Geometry check sheet. Reference: the model listing, model coordinates, mm. Face numbers are marked on the shaded views. A direction names the side the tool comes from. Round coordinates to 2 decimals unless told otherwise and drop trailing zeros. Write each loop counter-clockwise with the first axis right and the second up, starting at its lowest first coordinate (ties: lowest second). Pieces come first, ordered by that corner, then holes. Notation, with made-up numbers: M 54,78 L 89,78 A20 ccw 89,91 Z; hole C -27,-5.75 d10. An arc over 180 degrees is marked long. One line per item, written item: value. Start each with the question number.
1. Depth check by flat-ended pin: P1, Ø4, axis at x = 0, y = 8.5, coming from the +Z side; P2, Ø2, axis at y = 5.5, z = 36, coming from the -X side; P3, Ø0.5, axis at y = 4, z = 1.5, coming from the +X side. Enter the tip coordinate at first touch or a pass-through.
2. Scan lines: probe 1 along Y at (x, z) = (0, 1.2); probe 2 along Y at (x, z) = (-9, 29); probe 3 along X at (y, z) = (-9.25, 37). Record each from-to range of solid material in increasing order. Write a range as [from, to].
3. Section check D-D (z = 4). Record the boundary of the cut face in (x, y).
4. Release check for a two-part mould opening along Z. For the marked faces 4, 5, 6 and 7 record: pulls with the +Z half, pulls with the -Z half, needs draft (parallel to the pull), parting line crosses it, or undercut.
5. Section check A-A (x = 16.5). Record the boundary of the cut face in (y, z), and give its area (3 significant figures).
6. Access from +Z, -Z, +X, -X, +Y, -Y to the whole of each face (thin tool, end or side, straight path). Record for the marked faces 1, 2 and 3.
7. Section check B-B (y = 8.5). Count the separate pieces of the cut face and the enclosed holes in it, and give its area (3 significant figures).
8. Section check C-C (z = 44). Record the boundary of the cut face in (x, y), and give its area (3 significant figures).
from build123d import *

# Parameters (mm, degrees)
SKETCH1_R                = 14
BOSS_EXTRUDE1_DEPTH      = 50
SKETCH5_W                = 28
SKETCH5_H                = 50.034880911
BOSS_EXTRUDE2_DEPTH      = 21
SKETCH2_R                = 12.791811967
CUT_EXTRUDE1_DEPTH       = 48
SKETCH3_R                = 4
CUT_EXTRUDE2_DEPTH       = 49
SKETCH4_R                = 1.5
CUT_EXTRUDE3_DEPTH       = 49
SKETCH6_R                = 12.79
CUT_EXTRUDE5_DEPTH       = 21
SKETCH7_W                = 28
SKETCH7_H                = 4.634699127
CUT_EXTRUDE6_DEPTH       = 53
SKETCH8_W                = 50.034880911
SKETCH8_H                = 3.58
BOSS_EXTRUDE3_DEPTH      = 5
SKETCH13_R               = 1.5
CUT_EXTRUDE7_DEPTH       = 5
SKETCH14_W               = 50.034880911
SKETCH14_H               = 3.58
BOSS_EXTRUDE4_DEPTH      = 5
SKETCH15_R               = 1.5
CUT_EXTRUDE8_DEPTH       = 5
FILLET1_R                = 1
FILLET2_R                = 1
CUT_EXTRUDE9_DEPTH       = 56.96706514
CUT_EXTRUDE9_DEPTH_BACK  = 56.96706514
SKETCH16_W               = 38
SKETCH16_H               = 1.79
CUT_EXTRUDE10_DEPTH      = 62.684104138
CUT_EXTRUDE10_DEPTH_BACK = 62.684104138
SKETCH19_W               = 32.670016371
SKETCH19_H               = 14
SKETCH19_H_2             = 12.785300873


with BuildPart() as part:
    # Sketch1 → Boss-Extrude1 (new body)
    with BuildSketch(Plane.XY):
        with Locations(Location((0, 0, 0), (0, 0, 180))):
            Circle(SKETCH1_R)
    extrude(amount=BOSS_EXTRUDE1_DEPTH)

    # Sketch5 → Boss-Extrude2 (add)
    with BuildSketch(Plane(origin=(0, 0, 0), x_dir=(1, 0, 0), z_dir=(0, 1, 0))):
        with Locations((0, -25.017440456)):
            Rectangle(SKETCH5_W, SKETCH5_H)
    extrude(amount=BOSS_EXTRUDE2_DEPTH)

    # Sketch2 → Cut-Extrude1 (cut)
    with BuildSketch(Plane.XY.offset(50)):
        Circle(SKETCH2_R)
    extrude(amount=-CUT_EXTRUDE1_DEPTH, mode=Mode.SUBTRACT)

    # Sketch3 → Cut-Extrude2 (cut)
    with BuildSketch(Plane(origin=(0, 0, 0), x_dir=(-1, 0, 0), z_dir=(0, 0, -1))):
        Circle(SKETCH3_R)
    extrude(amount=-CUT_EXTRUDE2_DEPTH, mode=Mode.SUBTRACT)

    # Sketch4 → Cut-Extrude3 (cut)
    with BuildSketch(Plane(origin=(0, 0, 0), x_dir=(-1, 0, 0), z_dir=(0, 0, -1))):
        with Locations((0, -8.5)):
            Circle(SKETCH4_R)
        with Locations((0, 8.5)):
            Circle(SKETCH4_R)
        with Locations((8.5, 0)):
            Circle(SKETCH4_R)
        with Locations((-8.5, 0)):
            Circle(SKETCH4_R)
    extrude(amount=-CUT_EXTRUDE3_DEPTH, mode=Mode.SUBTRACT)

    # Sketch6 → Cut-Extrude5 (cut)
    with BuildSketch(Plane.XY.offset(50.034880911)):
        Circle(SKETCH6_R)
    extrude(amount=-CUT_EXTRUDE5_DEPTH, mode=Mode.SUBTRACT)

    # Sketch7 → Cut-Extrude6 (cut)
    with BuildSketch(Plane.XY.offset(50.034880911)):
        with Locations((0, 18.682650437)):
            Rectangle(SKETCH7_W, SKETCH7_H)
    extrude(amount=-CUT_EXTRUDE6_DEPTH, mode=Mode.SUBTRACT)

    # Sketch8 → Boss-Extrude3 (add)
    with BuildSketch(Plane(origin=(14, 0, 0), x_dir=(0, 0, -1), z_dir=(1, 0, 0))):
        with Locations((-25.017440456, 14.575300873)):
            Rectangle(SKETCH8_W, SKETCH8_H)
    extrude(amount=BOSS_EXTRUDE3_DEPTH)

    # Sketch13 → Cut-Extrude7 (cut)
    with BuildSketch(Plane.XZ.offset(-12.785300873)):
        with Locations(Location((16.5, 37.526160683, 0), (0, 0, 270))):
            Circle(SKETCH13_R)
        with Locations(Location((16.5, 12.508720228, 0), (0, 0, 270))):
            Circle(SKETCH13_R)
    extrude(amount=-CUT_EXTRUDE7_DEPTH, mode=Mode.SUBTRACT)

    # Sketch14 → Boss-Extrude4 (add)
    with BuildSketch(Plane.ZY.offset(14)):
        with Locations((25.017440456, 14.575300873)):
            Rectangle(SKETCH14_W, SKETCH14_H)
    extrude(amount=BOSS_EXTRUDE4_DEPTH)

    # Sketch15 → Cut-Extrude8 (cut)
    with BuildSketch(Plane.XZ.offset(-12.785300873)):
        with Locations(Location((-16.5, 12.508720228, 0), (0, 0, 270))):
            Circle(SKETCH15_R)
        with Locations(Location((-16.5, 37.526160683, 0), (0, 0, 270))):
            Circle(SKETCH15_R)
    extrude(amount=-CUT_EXTRUDE8_DEPTH, mode=Mode.SUBTRACT)

    # Fillet1
    fillet1_edges = [part.edges().sort_by_distance(p)[0] for p in [
        (10, 0, 0),
    ]]
    fillet(fillet1_edges, radius=FILLET1_R)

    # Fillet2
    fillet2_edges = [part.edges().sort_by_distance(p)[0] for p in [
        (1.5, -8.5, 0),
        (1.5, 8.5, 0),
        (-7, 0, 0),
    ]]
    fillet(fillet2_edges, radius=FILLET2_R)

    # Sketch16 → Cut-Extrude9 (cut, two sides: drawn at the far end of the back side and taken through both)
    with BuildSketch(Plane(origin=(0, 0, 0), x_dir=(-1, 0, 0), z_dir=(0, 0, -1)).offset(-CUT_EXTRUDE9_DEPTH_BACK)):
        with Locations((0, 15.470300873)):
            Rectangle(SKETCH16_W, SKETCH16_H)
    extrude(amount=CUT_EXTRUDE9_DEPTH + CUT_EXTRUDE9_DEPTH_BACK, mode=Mode.SUBTRACT)

    # Sketch19 → Cut-Extrude10 (cut, two sides: drawn at the far end of the back side and taken through both)
    with BuildSketch(Plane(origin=(14, 0, 0), x_dir=(0, 0, -1), z_dir=(1, 0, 0)).offset(-CUT_EXTRUDE10_DEPTH_BACK)):
        with Locations((-18.125008186, -7)):
            Rectangle(SKETCH19_W, SKETCH19_H)
        with Locations((-18.125008186, 6.392650437)):
            Rectangle(SKETCH19_W, SKETCH19_H_2)
    extrude(amount=CUT_EXTRUDE10_DEPTH + CUT_EXTRUDE10_DEPTH_BACK, mode=Mode.SUBTRACT)


solid = part.part
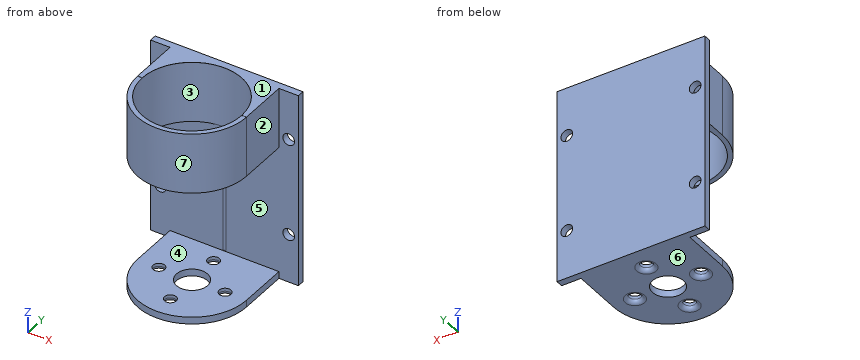
Result sheet:
1. P1: stops at z = 1.79
1. P2: stops at x = -14
1. P3: stops at x = 14
2. probe 1: y = [-14, -10], [-7, -4], [4, 7], [10, 14.58]
2. probe 2: y = [12.79, 14.58]
2. probe 3: x = [-10.51, -8.84], [8.84, 10.51]
3. outline: M -19,12.79 L -0.41,12.79 A12.79 cw 0.41,12.79 L 19,12.79 L 19,14.58 L -19,14.58 Z
4. face 4: undercut
4. face 5: undercut
4. face 6: pulls with the -Z half
4. face 7: needs draft
5. outline: M 12.79,0 L 14.58,0 L 14.58,11.01 L 12.79,11.01 Z; M 12.79,14.01 L 14.58,14.01 L 14.58,36.03 L 12.79,36.03 Z; M 12.79,39.03 L 14.58,39.03 L 14.58,50.03 L 12.79,50.03 Z
5. area: 78.8 mm2
6. face 1: +Z, +X, -X, +Y, -Y
6. face 2: +Z, -Z, +X, -Y
6. face 3: +Z
7. separate pieces: 4
7. enclosed holes: 0
7. area: 183 mm2
8. outline: M -19,12.79 L -14,12.79 L -14,0 A14 ccw 14,0 L 14,12.79 L 19,12.79 L 19,14.58 L -19,14.58 Z; hole C 0,0 d25.58
8. area: 220 mm2
